Geometry check sheet. Reference: the model listing, model coordinates, mm. Face numbers are marked on the shaded views. Coordinates: 2 decimals unless noted, no trailing zeros. Write each loop counter-clockwise with the first axis right and the second up, starting at its lowest first coordinate (ties: lowest second). Pieces come first, ordered by that corner, then holes. Notation, with made-up numbers: M 62.25,86.25 L 93.25,86.25 A35 cw 93.25,124.25 Z; hole C 20.5,54.25 d5. An arc over 180 degrees is marked long. Write each question's results on one line, items separated by ' | '.
```python
from build123d import *

# Parameters (mm, degrees)
SKETCH1_W               = 38.1
SKETCH1_H               = 38.1
SKETCH1_W_2             = 31.75
SKETCH1_H_2             = 31.75
BOSS_EXTRUDE1_DEPTH     = 176.2125
FILLET1_R               = 3.81
FILLET2_R               = 0.635
SKETCH2_R               = 3.2639
CUT_EXTRUDE1_DEPTH      = 1
CUT_EXTRUDE1_DEPTH_BACK = 39.1
SKETCH5_R               = 3.175
CUT_EXTRUDE3_DEPTH      = 39.1


with BuildPart() as part:
    # Sketch1 → Boss-Extrude1 (new body, symmetric)
    with BuildSketch(Plane(origin=(0, 0, 0), x_dir=(1, 0, 0), z_dir=(0, 1, 0))):
        Rectangle(SKETCH1_W, SKETCH1_H)
        Rectangle(SKETCH1_W_2, SKETCH1_H_2, mode=Mode.SUBTRACT)
    extrude(amount=BOSS_EXTRUDE1_DEPTH, both=True)

    # Fillet1
    fillet1_edges = [part.edges().sort_by_distance(p)[0] for p in [
        (19.05, 0, 19.05),
        (-19.05, 0, 19.05),
        (-19.05, 0, -19.05),
        (19.05, 0, -19.05),
    ]]
    fillet(fillet1_edges, radius=FILLET1_R)

    # Fillet2
    fillet2_edges = [part.edges().sort_by_distance(p)[0] for p in [
        (15.875, 0, -15.875),
        (-15.875, 0, -15.875),
        (-15.875, 0, 15.875),
        (15.875, 0, 15.875),
    ]]
    fillet(fillet2_edges, radius=FILLET2_R)

    # Sketch2 → Cut-Extrude1 (cut, two sides)
    with BuildSketch(Plane.XY.offset(19.05)) as cut_extrude1_sk:
        with Locations((0, 157.1625)):
            Circle(SKETCH2_R)
        with Locations((0, 104.1625)):
            Circle(SKETCH2_R)
        with Locations((0, 51.1625)):
            Circle(SKETCH2_R)
    extrude(amount=CUT_EXTRUDE1_DEPTH, mode=Mode.SUBTRACT)
    extrude(cut_extrude1_sk.sketch, amount=-CUT_EXTRUDE1_DEPTH_BACK, mode=Mode.SUBTRACT)

    # Sketch5 → Cut-Extrude3 (cut, through all)
    with BuildSketch(Plane(origin=(19.05, 0, 0), x_dir=(0, 0, -1), z_dir=(1, 0, 0))):
        with Locations((-10.05, -151.6875)):
            Circle(SKETCH5_R)
        with Locations((-10.05, -24.4875)):
            Circle(SKETCH5_R)
        with Locations((-10.05, -105.4875)):
            Circle(SKETCH5_R)
        with Locations((-10.05, -64.9875)):
            Circle(SKETCH5_R)
        with Locations((10.05, -151.6875)):
            Circle(SKETCH5_R)
        with Locations((10.05, -24.4875)):
            Circle(SKETCH5_R)
        with Locations((10.05, -105.4875)):
            Circle(SKETCH5_R)
        with Locations((10.05, -64.9875)):
            Circle(SKETCH5_R)
    extrude(amount=-CUT_EXTRUDE3_DEPTH, mode=Mode.SUBTRACT)


solid = part.part
```
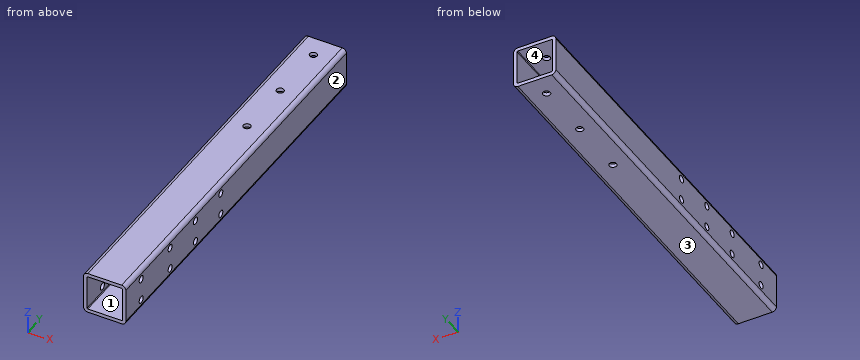
Q1. Mould release check, pull along Z, two halves, no side actions. Record for the marked faces 1, 2, 3 and 4: pulls with the +Z half, pulls with the -Z half, needs draft (parallel to the pull), parting line crosses it, or undercut.
Geometry check:
face 1: undercut | face 2: needs draft | face 3: pulls with the -Z half | face 4: undercut
Q2. Scan lines: probe 1 along Y at (x, z) = (0, -17); probe 2 along Y at (x, z) = (18.1, 10.05); probe 3 along Z at (x, y) = (6, -37) (3 decimals). Record each from-to range of solid material in increasing order.
Geometry check:
probe 1: y = -176.21 to 47.9, 54.43 to 100.9, 107.43 to 153.9, 160.43 to 176.21 | probe 2: y = -176.21 to -154.86, -148.51 to -108.66, -102.31 to -68.16, -61.81 to -27.66, -21.31 to 176.21 | probe 3: z = -19.05 to -15.875, 15.875 to 19.05
Q3. Sectioned sample at C-C on y = -18. Record the cut outline in (x, z) (3 decimals).
Geometry check:
outline: M -19.05,-15.24 A3.81 ccw -15.24,-19.05 L 15.24,-19.05 A3.81 ccw 19.05,-15.24 L 19.05,15.24 A3.81 ccw 15.24,19.05 L -15.24,19.05 A3.81 ccw -19.05,15.24 Z; hole M -15.875,-15.24 A0.635 ccw -15.24,-15.875 L 15.24,-15.875 A0.635 ccw 15.875,-15.24 L 15.875,15.24 A0.635 ccw 15.24,15.875 L -15.24,15.875 A0.635 ccw -15.875,15.24 Z
